Geometry: see drawing. Coordinates: mm, zero at the bounding-box minimum. Coordinates: 2 decimals unless noted, no trailing zeros. Loops run counter-clockwise (first coordinate to the right, second up) from the corner with the lowest first, then second, coordinate; pieces in that order, holes last. Notation, with made-up numbers: (53.25, 1.25) - (95.25, 1.25) arc R29 cw to (95.25, 34.25) - close; hole circle Ø11 at (73, -33). An arc over 180 degrees is marked (long way). Use a Markdown table: item, result. Add a question column.
1. Draft query along X for the marked faces 1, 2 and 3. Return one class per face: released by +X, released by -X, zero draft, split by the parting line, or undercut.
2. Section query B-B on y = 377. Return the cut outline in (x, z).
3. Section query C-C on x = 396. Return the cut outline in (y, z).
4. Section query D-D on y = 167.5. Return the cut outline in (x, z), then the cut area to 3 significant figures.
5. Section query A-A on z = 27. Return the cut outline in (x, y).
6. Contact query for flat-ended pins moving along their axis: P1, Ø6, axis at x = 267.5, z = 60.5, coming from the -Y side; P2, Ø2, axis at y = 627, z = 44, coming from the -X side; P3, Ø3, axis at y = 432.5, z = 25, coming from the -X side. Output: stop coordinate, or through.
7. Ray query, L1, parallel to Y at x = 447, z = 16.5; L2, parallel to X at y = 532, z = 38.5 (1 decimal); L3, parallel to X at y = 612, z = 33 (1 decimal). Return the intervals inside material, ascending. Write a range as [from, to].
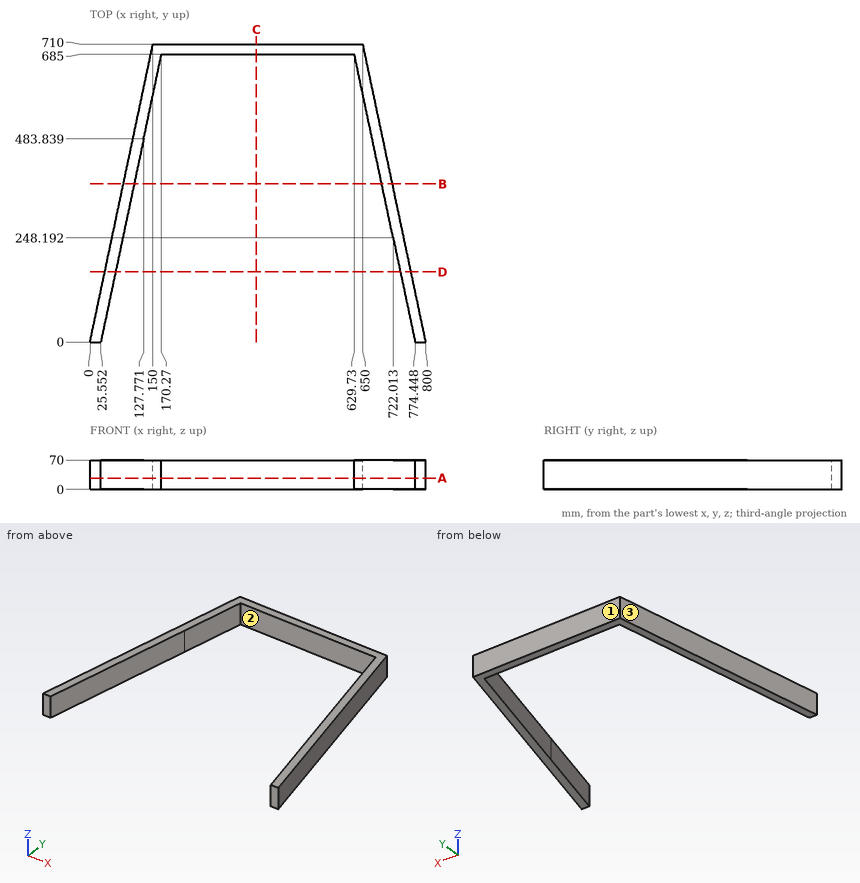
Resolved:
| question | item | result |
|---|---|---|
| 1 | face 1 | zero draft |
| 1 | face 2 | undercut |
| 1 | face 3 | released by -X |
| 2 | outline | (79.65, 0) - (105.2, 0) - (105.2, 70) - (79.65, 70) - close; (694.8, 0) - (720.35, 0) - (720.35, 70) - (694.8, 70) - close |
| 3 | outline | (685, 0) - (710, 0) - (710, 70) - (685, 70) - close |
| 4 | outline | (35.39, 0) - (60.94, 0) - (60.94, 70) - (35.39, 70) - close; (739.06, 0) - (764.61, 0) - (764.61, 70) - (739.06, 70) - close |
| 4 | area | 3,580 mm² |
| 5 | outline | (0, 0) - (25.55, 0) - (127.77, 483.84) - (170.27, 685) - (629.73, 685) - (722.01, 248.19) - (774.45, 0) - (800, 0) - (650, 710) - (150, 710) - close |
| 6 | P1 | y = 685 |
| 6 | P2 | x = 132.25 |
| 6 | P3 | x = 91.06 |
| 7 | L1 | [685, 710] |
| 7 | L2 | [112.4, 137.9], [662.1, 687.6] |
| 7 | L3 | [129.3, 154.8], [645.2, 670.7] |
